from build123d import *

# Parameters (mm, degrees)
SKETCH1_W                       = 87.884
SKETCH1_H                       = 94.488
BOSS_EXTRUDE1_DEPTH             = 139.446
SKETCH2_R                       = 8.5
BOSS_EXTRUDE2_DEPTH             = 55.118
SKETCH3_R                       = 39.6875
BOSS_EXTRUDE3_DEPTH             = 176.022
SKETCH4_W                       = 87.884
SKETCH4_H                       = 24.892
BOSS_EXTRUDE4_DEPTH             = 21.844
BOSS_EXTRUDE5_DEPTH             = 5.842
NOT_VERIFIED_EXTRUDE_DEPTH      = 10.033
SKETCH8_R                       = 2.75
CUT_EXTRUDE2_DEPTH              = 25.4
SKETCH7_R                       = 12.7
CHANGE_FOR_OPPOSITE_MOTOR_DEPTH = 339.432482365
SKETCH9_R                       = 3
CUT_EXTRUDE3_DEPTH              = 12.7
SKETCH10_R                      = 8.5725
BOSS_EXTRUDE6_DEPTH             = 6.096
SKETCH11_R                      = 1.5
CUT_EXTRUDE4_DEPTH              = 25.4
BOSS_EXTRUDE7_START             = 9.398
SKETCH12_R                      = 8.5
BOSS_EXTRUDE7_DEPTH             = 9.398
SKETCH13_R                      = 21.02690679
BOSS_EXTRUDE8_DEPTH             = 50.00625
SKETCH15_W                      = 14.986
SKETCH15_H                      = 14.986
BOSS_EXTRUDE9_DEPTH             = 6.35
BRAKE_AND_END_CAP_DEPTH         = 27.686
BRAKE_AND_END_CAP_DEPTH_BACK    = 9.398
SKETCH14_R                      = 41.275


with BuildPart() as part:
    # Sketch1 → Boss-Extrude1 (new body)
    with BuildSketch(Plane.XY):
        Rectangle(SKETCH1_W, SKETCH1_H)
    extrude(amount=-BOSS_EXTRUDE1_DEPTH)

    # Sketch2 → Boss-Extrude2 (add)
    with BuildSketch(Plane(origin=(-43.942, 0, 0), x_dir=(0, 0, -1), z_dir=(1, 0, 0))):
        with Locations(Location((41.91, 5.6388, 0), (0, 0, 90))):
            Circle(SKETCH2_R)
    extrude(amount=-BOSS_EXTRUDE2_DEPTH)

    # Sketch3 → Boss-Extrude3 (add)
    with BuildSketch(Plane(origin=(0, 0, -139.446), x_dir=(-1, 0, 0), z_dir=(0, 0, -1))):
        with Locations(Location((0, 27.686, 0), (0, 0, 150.475215814))):
            Circle(SKETCH3_R)
    extrude(amount=BOSS_EXTRUDE3_DEPTH)

    # Sketch4 → Boss-Extrude4 (add)
    with BuildSketch(Plane.XY.offset(-139.446)):
        with Locations((0, 59.69)):
            Rectangle(SKETCH4_W, SKETCH4_H)
    extrude(amount=BOSS_EXTRUDE4_DEPTH)

    # Sketch5 → Boss-Extrude5 (add, symmetric)
    with BuildSketch(Plane(origin=(0, 0, 0), x_dir=(0, 0, -1), z_dir=(1, 0, 0))):
        Polygon((41.00062989, 47.244), (117.602, 68.118364724), (117.602, 47.244), align=None)
    extrude(amount=BOSS_EXTRUDE5_DEPTH, both=True)

    # Sketch6 → not verified extrude (add)
    with BuildSketch(Plane(origin=(-43.942, 0, 0), x_dir=(0, 0, -1), z_dir=(1, 0, 0))):
        with BuildLine():
            Line((67.062792106, 10.685062506), (77.582823134, 7.605402716))
            ThreePointArc((77.582823134, 7.605402716), (103.428106849, -7.84112489), (73.318774576, -7.88601899))
            Line((73.318774576, -7.88601899), (62.51780348, -9.640144719))
            ThreePointArc((62.51780348, -9.640144719), (16.874294712, 11.237119098), (67.062792106, 10.685062506))
        make_face()
    extrude(amount=-NOT_VERIFIED_EXTRUDE_DEPTH)

    # Sketch8 → Cut-Extrude2 (cut)
    with BuildSketch(Plane(origin=(0, 0, -139.446), x_dir=(-1, 0, 0), z_dir=(0, 0, -1))):
        with Locations((-35.56, 63.246)):
            Circle(SKETCH8_R)
        with Locations((35.56, 63.246)):
            Circle(SKETCH8_R)
        with Locations((35.56, -7.874)):
            Circle(SKETCH8_R)
        with Locations((-35.56, -7.874)):
            Circle(SKETCH8_R)
    extrude(amount=-CUT_EXTRUDE2_DEPTH, mode=Mode.SUBTRACT)

    # Sketch7 → change for opposite motor (cut, through all)
    with BuildSketch(Plane.XY):
        with Locations((-14.097, -47.244)):
            Circle(SKETCH7_R)
    extrude(amount=-CHANGE_FOR_OPPOSITE_MOTOR_DEPTH, mode=Mode.SUBTRACT)

    # Sketch9 → Cut-Extrude3 (cut)
    with BuildSketch(Plane.XZ.offset(47.244)):
        with Locations((8.001, -7.9756)):
            Circle(SKETCH9_R)
        with Locations((8.001, -68.3768)):
            Circle(SKETCH9_R)
        with Locations((8.001, -128.778)):
            Circle(SKETCH9_R)
        with Locations((-36.449, -128.778)):
            Circle(SKETCH9_R)
        with Locations((-36.449, -68.3768)):
            Circle(SKETCH9_R)
        with Locations((-36.449, -7.9756)):
            Circle(SKETCH9_R)
    extrude(amount=-CUT_EXTRUDE3_DEPTH, mode=Mode.SUBTRACT)

    # Sketch10 → Boss-Extrude6 (add)
    with BuildSketch(Plane.XZ.offset(47.244)):
        with Locations(Location((32.639, -31.496, 0), (0, 0, 180))):
            Circle(SKETCH10_R)
        with Locations(Location((32.639, -104.4448, 0), (0, 0, 180))):
            Circle(SKETCH10_R)
    extrude(amount=BOSS_EXTRUDE6_DEPTH)

    # Sketch11 → Cut-Extrude4 (cut)
    with BuildSketch(Plane(origin=(0, 0, -315.468), x_dir=(-1, 0, 0), z_dir=(0, 0, -1))):
        with Locations(Location((-26.5, 27.686, 0), (0, 0, 90))):
            Circle(SKETCH11_R)
        with Locations(Location((26.5, 27.686, 0), (0, 0, 90))):
            Circle(SKETCH11_R)
    extrude(amount=-CUT_EXTRUDE4_DEPTH, mode=Mode.SUBTRACT)

    # Sketch12 → Boss-Extrude7 (add)
    with BuildSketch(Plane(origin=(43.942, 0, 0), x_dir=(0, 0, -1), z_dir=(1, 0, 0)).offset(BOSS_EXTRUDE7_START)):
        with BuildLine():
            Line((77.582823134, 7.605402716), (67.062792106, 10.685062506))
            ThreePointArc((67.062792106, 10.685062506), (16.874294712, 11.237119098), (62.51780348, -9.640144719))
            Line((62.51780348, -9.640144719), (73.318774576, -7.88601899))
            ThreePointArc((73.318774576, -7.88601899), (103.428106849, -7.84112489), (77.582823134, 7.605402716))
        make_face()
        with Locations(Location((41.91, 5.6388, 0), (0, 0, 90))):
            Circle(SKETCH12_R, mode=Mode.SUBTRACT)
    extrude(amount=-BOSS_EXTRUDE7_DEPTH)

    # Sketch13 → Boss-Extrude8 (add, symmetric)
    with BuildSketch(Plane(origin=(0, 0, 0), x_dir=(0, 0, -1), z_dir=(1, 0, 0))):
        with Locations(Location((278.212507153, 26.972524542, 0), (0, 0, 180))):
            Circle(SKETCH13_R)
    extrude(amount=BOSS_EXTRUDE8_DEPTH, both=True)

    # Sketch15 → Boss-Extrude9 (add)
    with BuildSketch(Plane(origin=(0, 0, -315.468), x_dir=(-1, 0, 0), z_dir=(0, 0, -1))):
        with Locations((0, 27.686)):
            Rectangle(SKETCH15_W, SKETCH15_H)
    extrude(amount=BOSS_EXTRUDE9_DEPTH)

    # Sketch14 → brake and end cap (add, two sides: drawn at the far end of the back side and taken through both)
    with BuildSketch(Plane(origin=(0, 0, -315.468), x_dir=(-1, 0, 0), z_dir=(0, 0, -1)).offset(-BRAKE_AND_END_CAP_DEPTH_BACK)):
        with Locations(Location((0, 27.686, 0), (0, 0, 90))):
            Circle(SKETCH14_R)
    extrude(amount=BRAKE_AND_END_CAP_DEPTH + BRAKE_AND_END_CAP_DEPTH_BACK)


solid = part.part
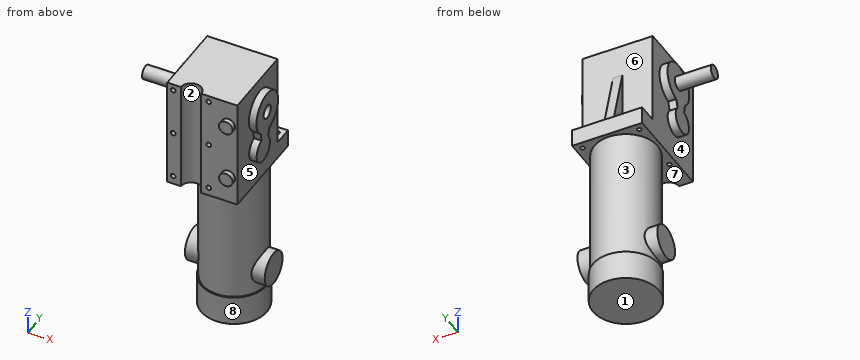
Can you work these out from the model? Positions are in its coordinate system, mm. Face numbers are marked on the shaded views. A direction names the side the tool comes from. Give positions to 0.01 mm unless a question says otherwise; leave off trailing zeros. Order: outer loops, then holes, each group sorted by start corner. A loop starts at its lowest first (then second) coordinate and runs counter-clockwise, first axis right, second up. Notation, with made-up numbers: (-34.5, 69.5) - (-21.5, 69.5) arc R23 cw to (-21.5, 107.5) - close; hole circle Ø6 at (28.25, 70.25). An arc over 180 degrees is marked (long way). Write each question's results on one line, items separated by ' | '.
1) Suppose I cut it at D-D, the plane y = 38. Write out the boundary of the cut face in (x, z), then the cut area to 3 significant figures.
Final values:
outline: (-50.01, -296.12) - (-38.32, -296.12) - (-38.32, -306.07) - (-39.97, -306.07) - (-39.97, -343.15) - (39.97, -343.15) - (39.97, -306.07) - (38.32, -306.07) - (38.32, -296.12) - (50.01, -296.12) - (50.01, -260.31) - (38.32, -260.31) - (38.32, -139.45) - (43.94, -139.45) - (43.94, 0) - (-43.94, 0) - (-43.94, -139.45) - (-38.32, -139.45) - (-38.32, -260.31) - (-50.01, -260.31) - close | area: 28,800 mm^2
2) Suppose I cut it at A-A, the plane y = -38. Write out the boundary of the cut face in (x, z).
Final values:
outline: (-43.94, -139.45) - (-22.81, -139.45) - (-22.81, 0) - (-43.94, 0) - close; (-5.39, -139.45) - (43.94, -139.45) - (43.94, 0) - (-5.39, 0) - close; hole circle Ø6 at (-36.45, -128.78); hole circle Ø6 at (-36.45, -68.38); hole circle Ø6 at (-36.45, -7.98); hole circle Ø6 at (8, -128.78); hole circle Ø6 at (8, -68.38); hole circle Ø6 at (8, -7.98)
3) On a 3-axis mill with a long thin cutter (end or side, diameter ignored), from which of +Z, -Z, +X, -X, +Y, -Y can I reach the whole of each face in a straight line? I mean the marked faces 4, 5, 6, 7 and 8. Say none if no direction works.
Final values:
face 4: -X | face 5: +X | face 6: +Z, +Y | face 7: none | face 8: -Z
4) Suppose I cut it at C-C, the plane z = -229. Write out the boundary of the cut face in (x, y) (1 decimal).
Final values:
outline: circle Ø79.4 at (0, 27.7)
5) If we mould it in two halves opening along X, with no side actions, what happens to the marked faces 1, 2 and 3? For each: pulls with the +X half, pulls with the -X half, needs draft (parallel to the pull), parting line crosses it, or undercut.
Final values:
face 1: needs draft | face 2: undercut | face 3: parting line crosses it
6) I'm going to push flat-ended pins straight in: pin 1 Ø21 at (y, z) = (24.5, -287) entering from +X; pin 2 Ø2.5 at (x, y) = (-26.5, 27.686) entering from +Z; pin 3 Ø3 at (x, z) = (19, -254) entering from -Y; pin 4 Ø9.5 at (x, z) = (8, -7.98) entering from -Y. Where does each tip first touch, or does it pass through?
Final values:
pin 1: stops at x = 50.01 | pin 2: stops at z = 0 | pin 3: stops at y = -7.93 | pin 4: stops at y = -47.24
7) Please list where these lines run through material, in increasing order: line 1 along Y through (x, z) = (-35.56, -128); line 2 along Y through (x, z) = (-35, -128); line 3 along X through (y, z) = (-14.5, -97) (3 decimals). Write a range as [from, to].
Final values:
line 1: y = [-34.54, -10.62], [-5.12, 60.5], [66, 72.14] | line 2: y = [-34.54, -10.57], [-5.18, 60.55], [65.94, 72.14] | line 3: x = [-53.975, 53.34]
8) Suppose I cut it at B-B, the plane y = 53.5. Write out the boundary of the cut face in (x, z).
Final values:
outline: (-43.94, -139.45) - (-30.15, -139.45) - (-30.15, -306.07) - (-32.21, -306.07) - (-32.21, -343.15) - (32.21, -343.15) - (32.21, -306.07) - (30.15, -306.07) - (30.15, -139.45) - (43.94, -139.45) - (43.94, -117.6) - (5.84, -117.6) - (5.84, -63.96) - (-5.84, -63.96) - (-5.84, -117.6) - (-43.94, -117.6) - close
